from build123d import *

# Parameters (mm, degrees)
SKETCH_1_R          = 3
EXTRUDE_1_DEPTH     = 6
SKETCH_1_4_R        = 1.9
CUT_EXTRUDE_1_DEPTH = 2
SKETCH_1_5_R        = 4.5
SKETCH_1_5_R_2      = 3
EXTRUDE_2_DEPTH     = 1
FILLET_1_R          = 1


with BuildPart() as part:
    # 草图1 → 凸台-拉伸1 (new body)
    with BuildSketch(Plane.XY):
        Circle(SKETCH_1_R)
    extrude(amount=EXTRUDE_1_DEPTH)

    # 草图1<4> → 切除-拉伸1 (cut)
    with BuildSketch(Plane.XY):
        Circle(SKETCH_1_4_R)
    extrude(amount=CUT_EXTRUDE_1_DEPTH, mode=Mode.SUBTRACT)

    # 草图1<5> → 凸台-拉伸2 (add)
    with BuildSketch(Plane.XY):
        Circle(SKETCH_1_5_R)
        Circle(SKETCH_1_5_R_2, mode=Mode.SUBTRACT)
    extrude(amount=EXTRUDE_2_DEPTH)

    # 圆角1
    fillet_1_edges = [part.edges().sort_by_distance(p)[0] for p in [
        (-3, 0, 6),
    ]]
    fillet(fillet_1_edges, radius=FILLET_1_R)


solid = part.part
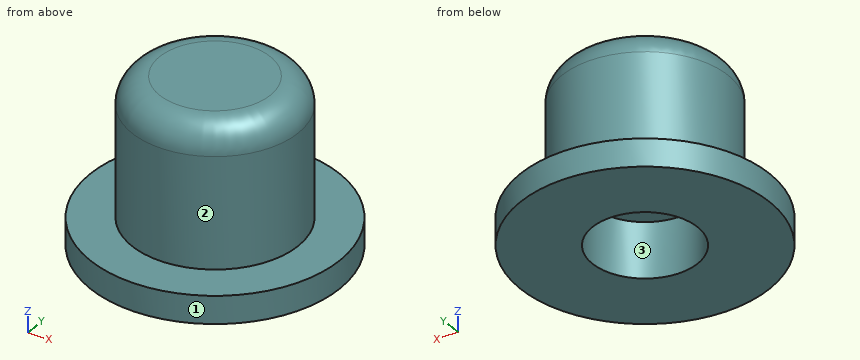
For this review, take the finished solid that the model builds, in its own axes (mm). Face numbers are marked on the shaded views. A direction names the side the tool comes from. Give positions to 0.01 mm unless a question says otherwise; leave off trailing zeros. Loops run counter-clockwise (first coordinate to the right, second up) from the corner with the lowest first, then second, coordinate; pieces in that order, holes last. Notation, with made-up numbers: (41, 51) - (89, 51) arc R29 cw to (89, 75) - close; hole circle Ø3 at (63.25, 23.5). An arc over 180 degrees is marked (long way). Write each question's results on one line, items separated by ' | '.
(1) For pin 1 Ø1.5 at (y, z) = (3, 1.5) entering from -X; pin 2 Ø1.5 at (x, z) = (1, 4.5) entering from -Y; pin 3 Ø3 at (y, z) = (2, 4) entering from +X, all flat-tipped, find the tip position at first contact; note any pin that passes through.
Conclusion:
pin 1: x = -3.78 | pin 2: y = -2.99 | pin 3: x = 2.96
(2) Take a section at D-D (y = 3.5). Give the boundary of the cut face in (x, z).
Conclusion:
outline: (-2.83, 0) - (2.83, 0) - (2.83, 1) - (-2.83, 1) - close
(3) For the marked faces 1, 2 and 3, list the 3-axis set-ups (+Z, -Z, +X, -X, +Y, -Y) from which the entire face can be reached by the end or side of a thin tool; tool diameter is ignored.
Conclusion:
face 1: +Z, -Z | face 2: +Z | face 3: -Z
(4) Take a section at C-C (z = 2.3). Give the boundary of the cut face in (x, y), then the cut area to 3 significant figures.
Conclusion:
outline: circle Ø6 at (0, 0) | area: 28.3 mm^2
(5) For line 1 along Z through (x, y) = (-0.75, 3); line 2 along Y through (x, z) = (0, 1.2); line 3 along Z through (x, y) = (0.75, 0.5), list the stretches that pass through material, from the lowest coordinate up.
Conclusion:
line 1: 0 to 1 | line 2: -3 to -1.9, 1.9 to 3 | line 3: 2 to 6
(6) Take a section at A-A (y = 0). Give the boundary of the cut face in (x, z), then the cut area to 3 significant figures.
Conclusion:
outline: (-4.5, 0) - (-1.9, 0) - (-1.9, 2) - (1.9, 2) - (1.9, 0) - (4.5, 0) - (4.5, 1) - (3, 1) - (3, 5) arc R1 ccw to (2, 6) - (-2, 6) arc R1 ccw to (-3, 5) - (-3, 1) - (-4.5, 1) - close | area: 31.0 mm^2
